```python
from build123d import *

# Parameters (mm, degrees)
SKETCH1_W           = 300
SKETCH1_H           = 180
BOSS_EXTRUDE1_DEPTH = 3
SKETCH2_W           = 40
SKETCH2_H           = 3
SKETCH2_W_2         = 3
SKETCH2_H_2         = 40
BOSS_EXTRUDE2_DEPTH = 3
SKETCH3_W           = 40
SKETCH3_H           = 3
CUT_EXTRUDE1_DEPTH  = 354.987287907
SKETCH4_W           = 40
SKETCH4_H           = 3
CUT_EXTRUDE2_DEPTH  = 3
SKETCH5_W           = 40
SKETCH5_H           = 3
CUT_EXTRUDE3_DEPTH  = 3
SKETCH6_W           = 40
SKETCH6_H           = 3
CUT_EXTRUDE4_DEPTH  = 3
SKETCH8_W           = 23.03
SKETCH8_H           = 12.59
CUT_EXTRUDE5_DEPTH  = 10
SKETCH9_R           = 1
CUT_EXTRUDE6_DEPTH  = 2
SKETCH12_R          = 1.5
CUT_EXTRUDE7_DEPTH  = 10
SKETCH13_R          = 1.5
CUT_EXTRUDE8_DEPTH  = 10


with BuildPart() as part:
    # Sketch1 → Boss-Extrude1 (new body)
    with BuildSketch(Plane(origin=(0, 0, 0), x_dir=(0, 0, -1), z_dir=(1, 0, 0))):
        with Locations((-150, 90)):
            Rectangle(SKETCH1_W, SKETCH1_H)
    extrude(amount=BOSS_EXTRUDE1_DEPTH)

    # Sketch2 → Boss-Extrude2 (add)
    with BuildSketch(Plane(origin=(3, 0, 0), x_dir=(0, 0, -1), z_dir=(1, 0, 0))):
        with Locations((-270, 181.5)):
            Rectangle(SKETCH2_W, SKETCH2_H)
        with Locations((-30, 181.5)):
            Rectangle(SKETCH2_W, SKETCH2_H)
        with Locations((1.5, 150)):
            Rectangle(SKETCH2_W_2, SKETCH2_H_2)
        with Locations((1.5, 30)):
            Rectangle(SKETCH2_W_2, SKETCH2_H_2)
        with Locations((-30, -1.5)):
            Rectangle(SKETCH2_W, SKETCH2_H)
        with Locations((-270, -1.5)):
            Rectangle(SKETCH2_W, SKETCH2_H)
        with Locations((-301.5, 150)):
            Rectangle(SKETCH2_W_2, SKETCH2_H_2)
        with Locations((-301.5, 30)):
            Rectangle(SKETCH2_W_2, SKETCH2_H_2)
    extrude(amount=-BOSS_EXTRUDE2_DEPTH)

    # Sketch3 → Cut-Extrude1 (cut, through all)
    with BuildSketch(Plane(origin=(3, 0, 0), x_dir=(0, 0, -1), z_dir=(1, 0, 0))):
        with Locations((-246, 162.5)):
            Rectangle(SKETCH3_W, SKETCH3_H)
    extrude(amount=-CUT_EXTRUDE1_DEPTH, mode=Mode.SUBTRACT)

    # Sketch4 → Cut-Extrude2 (cut)
    with BuildSketch(Plane(origin=(3, 0, 0), x_dir=(0, 0, -1), z_dir=(1, 0, 0))):
        with Locations((-54, 162.5)):
            Rectangle(SKETCH4_W, SKETCH4_H)
    extrude(amount=-CUT_EXTRUDE2_DEPTH, mode=Mode.SUBTRACT)

    # Sketch5 → Cut-Extrude3 (cut)
    with BuildSketch(Plane(origin=(3, 0, 0), x_dir=(0, 0, -1), z_dir=(1, 0, 0))):
        with Locations((-246, 17.5)):
            Rectangle(SKETCH5_W, SKETCH5_H)
    extrude(amount=-CUT_EXTRUDE3_DEPTH, mode=Mode.SUBTRACT)

    # Sketch6 → Cut-Extrude4 (cut)
    with BuildSketch(Plane(origin=(3, 0, 0), x_dir=(0, 0, -1), z_dir=(1, 0, 0))):
        with Locations((-54, 17.5)):
            Rectangle(SKETCH6_W, SKETCH6_H)
    extrude(amount=-CUT_EXTRUDE4_DEPTH, mode=Mode.SUBTRACT)

    # Sketch8 → Cut-Extrude5 (cut)
    with BuildSketch(Plane(origin=(3, 0, 0), x_dir=(0, 0, -1), z_dir=(1, 0, 0))):
        with Locations((-246, 90)):
            Rectangle(SKETCH8_W, SKETCH8_H)
    extrude(amount=-CUT_EXTRUDE5_DEPTH, mode=Mode.SUBTRACT)

    # Sketch9 → Cut-Extrude6 (cut)
    with BuildSketch(Plane(origin=(3, 0, 0), x_dir=(0, 0, -1), z_dir=(1, 0, 0))):
        with Locations((-260.015, 90)):
            Circle(SKETCH9_R)
        with Locations((-231.985, 90)):
            Circle(SKETCH9_R)
    extrude(amount=-CUT_EXTRUDE6_DEPTH, mode=Mode.SUBTRACT)

    # Sketch12 → Cut-Extrude7 (cut)
    with BuildSketch(Plane(origin=(1, 0, 0), x_dir=(0, 0, -1), z_dir=(1, 0, 0))):
        with Locations((-260.015, 90)):
            Circle(SKETCH12_R)
    extrude(amount=-CUT_EXTRUDE7_DEPTH, mode=Mode.SUBTRACT)

    # Sketch13 → Cut-Extrude8 (cut)
    with BuildSketch(Plane(origin=(1, 0, 0), x_dir=(0, 0, -1), z_dir=(1, 0, 0))):
        with Locations((-231.985, 90)):
            Circle(SKETCH13_R)
    extrude(amount=-CUT_EXTRUDE8_DEPTH, mode=Mode.SUBTRACT)


solid = part.part
```
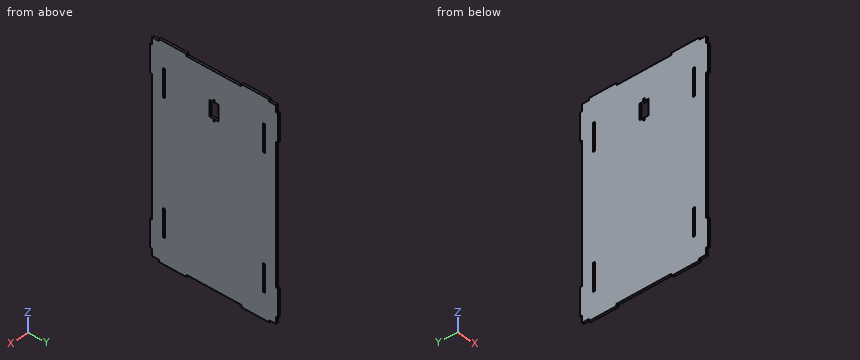
Can you work these out from the model? Positions are in its coordinate system, mm. Coordinates: 2 decimals unless noted, no trailing zeros. Write each loop counter-clockwise with the first axis right and the second up, starting at its lowest first coordinate (ties: lowest second). Pieces come first, ordered by that corner, then holes. Notation, with made-up numbers: M -34,19 L 8,19 A10 ccw 8,35 Z; hole C -31,14 d10. An arc over 180 degrees is marked long. Write item = value, one per line. Start each with the question number.
Q1. If I drill on L1, parallel to Z at x = 0.8, y = 90 (3 decimals); L2, parallel to Y at x = 2, z = 54; L3, parallel to Z at x = 2.35, y = 90 (3 decimals), over which ranges is the centre line in solid material (lowest first)? Write a range as [from, to].
Q2. I'm going to push flat-ended pins straight in: pin 1 (1.5 mm diameter, centred on x = 2.5, z = 103, fed in from +Y); pin 2 (1.5 mm diameter, centred on x = 2, y = 87, fed in from +Z); pin 3 (1.5 mm diameter, centred on y = 90.5, z = 260, fed in from -X). Where does each tip first touch, or does it pass through?
Q3. If we section it at B-B, the plane y = 101: Write out the boundary of the cut face in (x, z).
Q4. If we section it at C-C, the plane z = 129: Write out the boundary of the cut face in (x, y).
Q5. If we section it at A-A, the plane x = 0.5: State how many separate pieces and enclosed holes the cut face has, then the cut area to 3 significant figures.
Check sheet entries:
q1.L1 = [0, 230.485], [233.485, 234.485], [257.515, 258.515], [261.515, 300]
q1.L2 = [0, 16], [19, 161], [164, 180]
q1.L3 = [0, 230.985], [232.985, 234.485], [257.515, 259.015], [261.015, 300]
q2.pin_1 = 180
q2.pin_2 = 300
q2.pin_3 = 1
q3.outline = M 0,0 L 3,0 L 3,300 L 0,300 Z
q4.outline = M 0,0 L 3,0 L 3,180 L 0,180 Z
q5.separate_pieces = 1
q5.enclosed_holes = 7
q5.area = 54,200 mm²
